The listing builds one solid part. Answer for the finished solid, in the listing's coordinates (mm). Face numbers are marked on the shaded views. A direction names the side the tool comes from. Coordinates: 2 decimals unless noted, no trailing zeros. Order: outer loops, then holes, each group sorted by start corner. A loop starts at its lowest first (then second) coordinate and runs counter-clockwise, first axis right, second up. Notation, with made-up numbers: M 60,46.5 L 68,46.5 A14 cw 68,66.5 Z; hole C 84,-1 d10. An arc over 180 degrees is marked long. One line per item, written item: value. Start each with the question number.
Q1. The part is cut by section C-C on y = 15. Give the vertices of the cut face in (x, z).
Q2. The part is cut by section D-D on z = 8.75. Give the vertices of the cut face in (x, y).
Q3. Each of these flat-tipped pins is pushed along its axis until it touches: pin 1 Ø3 at (y, z) = (15, 0) entering from -X; pin 2 Ø4.5 at (x, y) = (0, 15) entering from -Z; pin 3 Ø2 at (x, y) = (-1, 13) entering from +Z; pin 4 Ø6 at (x, z) = (-7.5, 1.5) entering from +Y. Where does it stop, or does it pass through?
Q4. For the marked faces 5, 6, 7 and 8, determine the directions among +Z, -Z, +X, -X, +Y, -Y from which every point of the face is accessible in a straight line to the end or side of a thin tool.
Q5. Determine the mould class of the marked faces 1, 2, 3 and 4 for opening direction Y: pulls with the +Y half, pulls with the -Y half, needs draft (parallel to the pull), parting line crosses it, or undercut.
Q6. The part is cut by section A-A on x = 0. Give the vertices of the cut face in (y, z), then the cut area to 3 significant figures.
Q7. Straight lines are drawn through the part: line 1 along Y through (x, z) = (7.5, -7.75); line 2 along X through (y, z) = (4.5, 0); line 3 along X through (y, z) = (11.75, 0). For each, find the intervals that lie inside material, in ascending order. Write a range as [from, to].
Q8. The part is cut by section B-B on z = 0. Give the vertices of the cut face in (x, y).
```python
from build123d import *

# Parameters (mm, degrees)
SKETCH1_R                = 7.83
BOSS_EXTRUDE1_DEPTH      = 10
CUT_EXTRUDE1_DEPTH       = 14.660812567
FILLET1_R                = 0.38
CIRPATTERN1_COUNT        = 10
FILLET1_OF_CIRPATTERN1_R = 0.38
SKETCH3_R                = 2.55
CUT_EXTRUDE2_DEPTH       = 15.840354998
SKETCH4_R                = 11
BOSS_EXTRUDE2_DEPTH      = 1
SKETCH5_R                = 11
BOSS_EXTRUDE3_DEPTH      = 1
SKETCH6_R                = 6
BOSS_EXTRUDE4_DEPTH      = 8
SKETCH7_R                = 2.55
CUT_EXTRUDE3_DEPTH       = 26.337718919
CUT_EXTRUDE3_DEPTH_BACK  = 26.337718919
M4_TAPPED_HOLE1_REACH    = 27.807
M4_TAPPED_HOLE1_BORE_R   = 1.65
M4_TAPPED_HOLE2_REACH    = 27.807
M4_TAPPED_HOLE2_BORE_R   = 1.65
CHAMFER1_SIZE            = 0.5


with BuildPart() as part:
    # Sketch1 → Boss-Extrude1 (new body)
    with BuildSketch(Plane(origin=(0, 0, 0), x_dir=(1, 0, 0), z_dir=(0, 1, 0))):
        with Locations(Location((0, 0, 0), (0, 0, 270))):
            Circle(SKETCH1_R)
    extrude(amount=BOSS_EXTRUDE1_DEPTH)

    # Sketch2 → Cut-Extrude1 (cut, symmetric)
    with BuildSketch(Plane(origin=(0, 2, 0), x_dir=(1, 0, 0), z_dir=(0, 1, 0))):
        with BuildLine():
            Line((-1.285, 7.7238381), (-0.723625557, 6.519966722))
            ThreePointArc((-0.723625557, 6.519966722), (0, 6.56), (0.723625557, 6.519966722))
            Line((0.723625557, 6.519966722), (1.285, 7.7238381))
            ThreePointArc((1.285, 7.7238381), (0, 7.83), (-1.285, 7.7238381))
        make_face()
    cut_extrude1 = extrude(amount=CUT_EXTRUDE1_DEPTH, both=True, mode=Mode.SUBTRACT)

    # Fillet1
    fillet1_edges = [part.edges().sort_by_distance(p)[0] for p in [
        (1.285, 5, -7.7238381),
        (0.723625557, 5, -6.519966722),
        (-0.723625557, 5, -6.519966722),
        (-1.285, 5, -7.7238381),
    ]]
    fillet(fillet1_edges, radius=FILLET1_R)

    # CirPattern1: Cut-Extrude1 ×10 about axis
    cirpattern1_axis = Axis((0, 0, 0), (0, 1, 0))
    for i in range(1, CIRPATTERN1_COUNT):
        add(cut_extrude1.rotate(cirpattern1_axis, i * 360 / CIRPATTERN1_COUNT), mode=Mode.SUBTRACT)

    # Fillet1 of CirPattern1
    fillet1_of_cirpattern1_edges = [part.edges().sort_by_distance(p)[0] for p in [
        (-3.500371289, 5, -7.004020334),
        (-3.246914912, 5, -5.700100311),
        (-4.417765658, 5, -4.84942745),
        (-5.579544964, 5, -5.493412236),
        (-6.948719718, 5, -3.608904858),
        (-5.977244242, 5, -2.702989321),
        (-6.424469431, 5, -1.326571719),
        (-7.742893394, 5, -1.164689611),
        (-7.742893394, 5, 1.164689611),
        (-6.424469431, 5, 1.326571719),
        (-5.977244242, 5, 2.702989321),
        (-6.948719718, 5, 3.608904858),
        (-5.579544964, 5, 5.493412236),
        (-4.417765658, 5, 4.84942745),
        (-3.246914912, 5, 5.700100311),
        (-3.500371289, 5, 7.004020334),
        (-1.285, 5, 7.7238381),
        (-0.723625557, 5, 6.519966722),
        (0.723625557, 5, 6.519966722),
        (1.285, 5, 7.7238381),
        (3.500371289, 5, 7.004020334),
        (3.246914912, 5, 5.700100311),
        (4.417765658, 5, 4.84942745),
        (5.579544964, 5, 5.493412236),
        (6.948719718, 5, 3.608904858),
        (5.977244242, 5, 2.702989321),
        (6.424469431, 5, 1.326571719),
        (7.742893394, 5, 1.164689611),
        (7.742893394, 5, -1.164689611),
        (6.424469431, 5, -1.326571719),
        (5.977244242, 5, -2.702989321),
        (6.948719718, 5, -3.608904858),
        (5.579544964, 5, -5.493412236),
        (4.417765658, 5, -4.84942745),
        (3.246914912, 5, -5.700100311),
        (3.500371289, 5, -7.004020334),
    ]]
    fillet(fillet1_of_cirpattern1_edges, radius=FILLET1_OF_CIRPATTERN1_R)

    # Sketch3 → Cut-Extrude2 (cut, through all)
    with BuildSketch(Plane(origin=(0, 10, 0), x_dir=(1, 0, 0), z_dir=(0, 1, 0))):
        with Locations(Location((0, 0, 0), (0, 0, 270))):
            Circle(SKETCH3_R)
    extrude(amount=-CUT_EXTRUDE2_DEPTH, mode=Mode.SUBTRACT)

    # Sketch4 → Boss-Extrude2 (add)
    with BuildSketch(Plane.XZ):
        with Locations(Location((0, 0, 0), (0, 0, 270))):
            Circle(SKETCH4_R)
    extrude(amount=BOSS_EXTRUDE2_DEPTH)

    # Sketch5 → Boss-Extrude3 (add)
    with BuildSketch(Plane(origin=(0, 10, 0), x_dir=(1, 0, 0), z_dir=(0, 1, 0))):
        with Locations(Location((0, 0, 0), (0, 0, 90))):
            Circle(SKETCH5_R)
    extrude(amount=BOSS_EXTRUDE3_DEPTH)

    # Sketch6 → Boss-Extrude4 (add)
    with BuildSketch(Plane(origin=(0, 11, 0), x_dir=(1, 0, 0), z_dir=(0, 1, 0))):
        with Locations(Location((0, 0, 0), (0, 0, 270))):
            Circle(SKETCH6_R)
    extrude(amount=BOSS_EXTRUDE4_DEPTH)

    # Sketch7 → Cut-Extrude3 (cut, two sides)
    with BuildSketch(Plane(origin=(0, 19, 0), x_dir=(1, 0, 0), z_dir=(0, 1, 0))) as cut_extrude3_sk:
        with Locations(Location((0, 0, 0), (0, 0, 270))):
            Circle(SKETCH7_R)
    extrude(amount=CUT_EXTRUDE3_DEPTH, mode=Mode.SUBTRACT)
    extrude(cut_extrude3_sk.sketch, amount=-CUT_EXTRUDE3_DEPTH_BACK, mode=Mode.SUBTRACT)

    # M4 Tapped Hole1 bore (on position points) → M4 Tapped Hole1 (cut, up to next)
    with BuildSketch(Plane(origin=(0, 15, -6), x_dir=(-1, 0, 0), z_dir=(0, 0, -1)), mode=Mode.PRIVATE) as m4_tapped_hole1_sk1:
        Circle(M4_TAPPED_HOLE1_BORE_R)
    m4_tapped_hole1_tool1 = extrude(m4_tapped_hole1_sk1.sketch, amount=-M4_TAPPED_HOLE1_REACH, mode=Mode.PRIVATE) & part.part
    add(m4_tapped_hole1_tool1.solids().sort_by_distance((0, 15, -6))[0], mode=Mode.SUBTRACT)

    # M4 Tapped Hole2 bore (on position points) → M4 Tapped Hole2 (cut, up to next)
    with BuildSketch(Plane(origin=(6, 15, 0), x_dir=(0, 0, 1), z_dir=(1, 0, 0)), mode=Mode.PRIVATE) as m4_tapped_hole2_sk1:
        Circle(M4_TAPPED_HOLE2_BORE_R)
    m4_tapped_hole2_tool1 = extrude(m4_tapped_hole2_sk1.sketch, amount=-M4_TAPPED_HOLE2_REACH, mode=Mode.PRIVATE) & part.part
    add(m4_tapped_hole2_tool1.solids().sort_by_distance((6, 15, 0))[0], mode=Mode.SUBTRACT)

    # Chamfer1
    chamfer1_edges = [part.edges().sort_by_distance(p)[0] for p in [
        (0, 19, -6),
    ]]
    chamfer(chamfer1_edges, length=CHAMFER1_SIZE)


solid = part.part
```
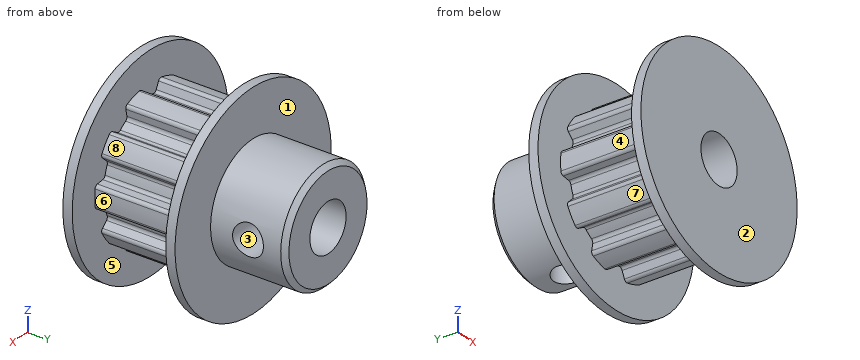
Output:
1. outline: M -1.65,-5.77 L -1.65,-1.94 A2.55 cw long 1.94,1.65 L 5.77,1.65 A6 ccw long Z; M 1.65,-5.77 A6 ccw 5.77,-1.65 L 1.94,-1.65 A2.55 cw 1.65,-1.94 Z
2. outline: M -6.67,-1 L 6.67,-1 L 6.67,0 L -6.67,0 Z; M -6.67,10 L 6.67,10 L 6.67,11 L -6.67,11 Z
3. pin 1: stops at x = -6
3. pin 2: stops at z = -6
3. pin 3: stops at z = 6
3. pin 4: stops at y = 19
4. face 5: none
4. face 6: +X
4. face 7: -Z, -X
4. face 8: +Z, +X
5. face 1: pulls with the +Y half
5. face 2: pulls with the -Y half
5. face 3: undercut
5. face 4: undercut
6. outline: M -1,-11 L 0,-11 L 0,-6.56 L 10,-6.56 L 10,-11 L 11,-11 L 11,-6 L 13.35,-6 L 13.35,-2.55 L -1,-2.55 Z; M -1,2.55 L 19,2.55 L 19,5.5 L 18.5,6 L 11,6 L 11,11 L 10,11 L 10,6.56 L 0,6.56 L 0,11 L -1,11 Z; M 16.65,-6 L 18.5,-6 L 19,-5.5 L 19,-2.55 L 16.65,-2.55 Z
6. area: 158 mm^2
7. line 1: y = [-1, 0], [10, 11]
7. line 2: x = [-7.83, -2.55], [2.55, 7.83]
7. line 3: x = [-6, -2.55], [2.55, 6]
8. outline: M -11,-1 L -2.55,-1 L -2.55,19 L -5.5,19 L -6,18.5 L -6,11 L -11,11 L -11,10 L -7.83,10 L -7.83,0 L -11,0 Z; M 2.55,-1 L 11,-1 L 11,0 L 7.83,0 L 7.83,10 L 11,10 L 11,11 L 6,11 L 6,13.35 L 2.55,13.35 Z; M 2.55,16.65 L 6,16.65 L 6,18.5 L 5.5,19 L 2.55,19 Z
